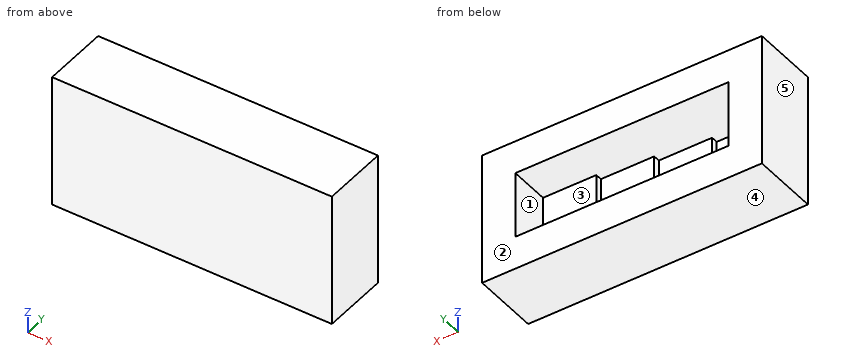
from build123d import *

# Parameters (mm, degrees)
BOSS_EXTRUDE1_DEPTH = 10
SKETCH6_W           = 10
SKETCH6_H           = 10
BOSS_EXTRUDE2_DEPTH = 5
SKETCH7_W           = 37
SKETCH7_H           = 10
BOSS_EXTRUDE3_DEPTH = 5
SKETCH8_W           = 15
SKETCH8_H           = 10
BOSS_EXTRUDE4_DEPTH = 5
SKETCH9_W           = 42
SKETCH9_H           = 10
BOSS_EXTRUDE5_DEPTH = 5


with BuildPart() as part:
    # Sketch3 → Boss-Extrude1 (new body)
    with BuildSketch(Plane.XY):
        Polygon((32, 4), (32, 0), (20, 0), (0, 0), (0, 1), (8, 1), (8, 2), (16, 2), (16, 3), (24, 3), (24, 4), align=None)
    extrude(amount=BOSS_EXTRUDE1_DEPTH)

    # Sketch6 → Boss-Extrude2 (add)
    with BuildSketch(Plane(origin=(0, 0, 0), x_dir=(0, 0, -1), z_dir=(1, 0, 0))):
        with Locations((-5, 5)):
            Rectangle(SKETCH6_W, SKETCH6_H)
    extrude(amount=-BOSS_EXTRUDE2_DEPTH)

    # Sketch7 → Boss-Extrude3 (add)
    with BuildSketch(Plane(origin=(0, 0, 0), x_dir=(-1, 0, 0), z_dir=(0, 0, -1))):
        with Locations((-13.5, 5)):
            Rectangle(SKETCH7_W, SKETCH7_H)
    extrude(amount=BOSS_EXTRUDE3_DEPTH)

    # Sketch8 → Boss-Extrude4 (add)
    with BuildSketch(Plane(origin=(32, 0, 0), x_dir=(0, 0, -1), z_dir=(1, 0, 0))):
        with Locations((-2.5, 5)):
            Rectangle(SKETCH8_W, SKETCH8_H)
    extrude(amount=BOSS_EXTRUDE4_DEPTH)

    # Sketch9 → Boss-Extrude5 (add)
    with BuildSketch(Plane.XY.offset(10)):
        with Locations((16, 5)):
            Rectangle(SKETCH9_W, SKETCH9_H)
    extrude(amount=BOSS_EXTRUDE5_DEPTH)


solid = part.part
Geometry: final body of the model. Coordinates: model frame, mm. Face numbers are marked on the shaded views. A direction names the side the tool comes from. Round coordinates to 2 decimals unless told otherwise and drop trailing zeros. Loops run counter-clockwise (first coordinate to the right, second up) from the corner with the lowest first, then second, coordinate; pieces in that order, holes last. Notation, with made-up numbers: (31, 10.5) -> (60, 10.5) arc R12 cw to (60, 23.5) -> close; hole circle Ø5 at (-11.75, 9). An arc over 180 degrees is marked (long way). One line per question, with ' | ' between items. Start each with the question number.
1. Section B-B on z = 4. Output: boundary loops of the cut face in (x, y), and give its area (3 significant figures).
2. Section C-C on x = 6.5. Output: boundary loops of the cut face in (y, z), and give its area (3 significant figures).
3. Section A-A on y = 8.5. Output: boundary loops of the cut face in (x, z), and give its area (3 significant figures).
4. Contact query for a flat-ended pin moving along its axis: pin 1 (6.5 mm diameter, centred on x = 5.5, z = 5.5, fed in from +Y). Output: stop coordinate, or through.
5. Mould query, pull axis X, two halves, no side actions, for the marked faces 3, 4 and 5. Classes: pulls with the +X half, pulls with the -X half, needs draft (parallel to the pull), parting line crosses it, or undercut.
6. Set-up query: the marked faces 1 and 2. Return all of +Z, -Z, +X, -X, +Y, -Y with unobstructed straight access to the full face (end or side cutting, diameter ignored); none if empty.
7. Line query: line 1 along X through (y, z) = (5.5, 5.25); line 2 along X through (y, z) = (3.25, 3); line 3 along Z through (x, y) = (24, 9). Output: solid intervals per line, ascending. Write a range as [from, to].
8. Section D-D on x = 18.5. Output: boundary loops of the cut face in (y, z), and give its area (3 significant figures).
Returned:
1) outline: (-5, 0) -> (37, 0) -> (37, 10) -> (32, 10) -> (32, 4) -> (24, 4) -> (24, 3) -> (16, 3) -> (16, 2) -> (8, 2) -> (8, 1) -> (0, 1) -> (0, 10) -> (-5, 10) -> close | area: 180 mm2
2) outline: (0, -5) -> (10, -5) -> (10, 0) -> (1, 0) -> (1, 10) -> (10, 10) -> (10, 15) -> (0, 15) -> close | area: 110 mm2
3) outline: (-5, -5) -> (37, -5) -> (37, 15) -> (-5, 15) -> close; hole (0, 0) -> (32, 0) -> (32, 10) -> (0, 10) -> close | area: 520 mm2
4) pin 1: stops at y = 2
5) face 3: undercut | face 4: needs draft | face 5: pulls with the -X half
6) face 1: +Y | face 2: +Z, -Z, +X, -X, +Y
7) line 1: x = [-5, 0], [32, 37] | line 2: x = [-5, 0], [24, 37] | line 3: z = [-5, 0], [10, 15]
8) outline: (0, -5) -> (10, -5) -> (10, 0) -> (3, 0) -> (3, 10) -> (10, 10) -> (10, 15) -> (0, 15) -> close | area: 130 mm2
